```python
from build123d import *

# Parameters (mm, degrees)
F0_R     = 1.5
F0_R_2   = 2.5
F1_DEPTH = 3


with BuildPart() as f1:
    # F0 (on Front) → F1 (new body)
    with BuildSketch(Plane.XZ):
        with BuildLine():
            ThreePointArc((-11.428203, -8.5), (-10.549524, -10.62132), (-8.428203, -11.5))
            Line((-8.428203, -11.5), (8.428203, -11.5))
            ThreePointArc((8.428203, -11.5), (10.549524, -10.62132), (11.428203, -8.5))
            Line((11.428203, -8.5), (11.428203, 8.5))
            ThreePointArc((11.428203, 8.5), (10.549524, 10.62132), (8.428203, 11.5))
            Line((8.428203, 11.5), (-8.428203, 11.5))
            ThreePointArc((-8.428203, 11.5), (-10.549524, 10.62132), (-11.428203, 8.5))
            Line((-11.428203, 8.5), (-11.428203, -8.5))
        make_face()
        with Locations((-6.928203, -7)):
            Circle(F0_R, mode=Mode.SUBTRACT)
        with Locations((0, -6)):
            Circle(F0_R_2, mode=Mode.SUBTRACT)
        with Locations((6.928203, -7)):
            Circle(F0_R, mode=Mode.SUBTRACT)
        with Locations((-6.928203, 7)):
            Circle(F0_R, mode=Mode.SUBTRACT)
        with Locations((0, 6)):
            Circle(F0_R_2, mode=Mode.SUBTRACT)
        with Locations((6.928203, 7)):
            Circle(F0_R, mode=Mode.SUBTRACT)
    extrude(amount=F1_DEPTH)


solid = f1.part
```
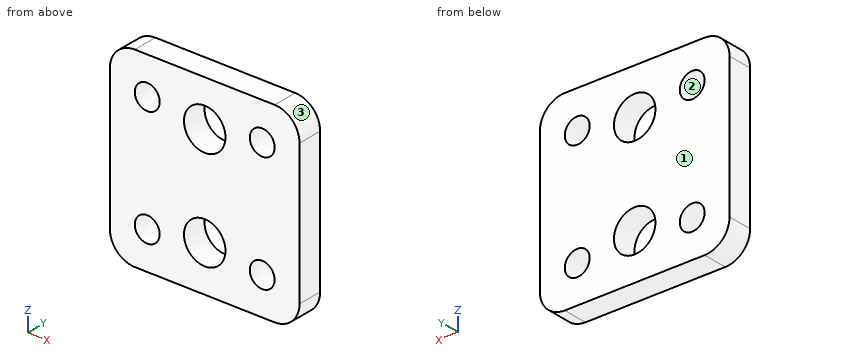
Build history of the part. All positions in model axes, mm. Face numbers are marked on the shaded views. Coordinates: 2 decimals unless noted, no trailing zeros. Order: outer loops, then holes, each group sorted by start corner. A loop starts at its lowest first (then second) coordinate and runs counter-clockwise, first axis right, second up. Notation, with made-up numbers: (81.25, 15.25) -> (131.25, 15.25) arc R23 cw to (131.25, 51.25) -> close; hole circle Ø9 at (39.5, 50.25). An arc over 180 degrees is marked (long way). Answer in a Markdown table with one row per item. Add a question column.
Q1. Band-saw the part on C-C, the plane y = -1.65. List the corners of the cut face in (x, z).
Q2. Band-saw the part on A-A, the plane x = 1.5. List the corners of the cut face in (y, z).
Q3. Band-saw the part on B-B, the plane z = 6. List the corners of the cut face in (x, y).
Q4. Wall check: line 1 along Z through (x, y) = (-7, -0.8); line 2 along Z through (x, y) = (0, -1.65); line 3 along X through (y, z) = (-2.25, 4.75). Give the ranges that are in metal, low to high. Write a range as [from, to].
Q5. Band-saw the part on D-D, the plane x = 7.25. List the corners of the cut face in (y, z), then the cut area to 3 significant figures.
Q6. Mould opens along Z. For the marked faces 1, 2 and 3 say: +Z half, -Z half, draft (parallel to the pull), parting line (faces both ways), or undercut.
Q7. Drop a flat-ended pin along its axis: pin 1 (3.5 mm diameter, centred on x = -6.93, z = -7, fed in from -Y). Give the stop position or say it passes through.
Answers follow:
| question | item | result |
|---|---|---|
| 1 | outline | (-11.43, -8.5) arc R3 ccw to (-8.43, -11.5) -> (8.43, -11.5) arc R3 ccw to (11.43, -8.5) -> (11.43, 8.5) arc R3 ccw to (8.43, 11.5) -> (-8.43, 11.5) arc R3 ccw to (-11.43, 8.5) -> close; hole circle Ø3 at (-6.93, -7); hole circle Ø3 at (-6.93, 7); hole circle Ø5 at (0, -6); hole circle Ø5 at (0, 6); hole circle Ø3 at (6.93, -7); hole circle Ø3 at (6.93, 7) |
| 2 | outline | (-3, -11.5) -> (0, -11.5) -> (0, -8) -> (-3, -8) -> close; (-3, -4) -> (0, -4) -> (0, 4) -> (-3, 4) -> close; (-3, 8) -> (0, 8) -> (0, 11.5) -> (-3, 11.5) -> close |
| 3 | outline | (-11.43, -3) -> (-8.05, -3) -> (-8.05, 0) -> (-11.43, 0) -> close; (-5.81, -3) -> (-2.5, -3) -> (-2.5, 0) -> (-5.81, 0) -> close; (2.5, -3) -> (5.81, -3) -> (5.81, 0) -> (2.5, 0) -> close; (8.05, -3) -> (11.43, -3) -> (11.43, 0) -> (8.05, 0) -> close |
| 4 | line 1 | [-11.5, -8.5], [-5.5, 5.5], [8.5, 11.5] |
| 4 | line 2 | [-11.5, -8.5], [-3.5, 3.5], [8.5, 11.5] |
| 4 | line 3 | [-11.43, -2.17], [2.17, 11.43] |
| 5 | outline | (-3, -11.5) -> (0, -11.5) -> (0, -8.47) -> (-3, -8.47) -> close; (-3, -5.53) -> (0, -5.53) -> (0, 5.53) -> (-3, 5.53) -> close; (-3, 8.47) -> (0, 8.47) -> (0, 11.5) -> (-3, 11.5) -> close |
| 5 | area | 51.4 mm^2 |
| 6 | face 1 | draft |
| 6 | face 2 | undercut |
| 6 | face 3 | +Z half |
| 7 | pin 1 | y = -3 |
